Read the model definition and answer for the solid it produces. Units are mm, in the model's axes. A direction names the side the tool comes from. Give positions to 0.01 mm unless a question says otherwise; leave off trailing zeros. Order: outer loops, then holes, each group sorted by start corner. A loop starts at its lowest first (then second) coordinate and runs counter-clockwise, first axis right, second up.
Item 1: A cutting plane is placed at A-A (y = 3.75). Write down the section's boundary in (x, z).
Item 2: Which of the six approach directions +Z, -Z, +X, -X, +Y, -Y give full straight-line access (tool end or side, diameter ignored) to faces 1 (the face through (5, 3, 3.6)), 2 (the face through (5, 12, 1))?
Item 3: The mould has two halves that part along X. Classify faces 3 (the face through (3.92, 2.96, 2.85)), 4 (the face through (0, 6.9, 0.6)), 5 (the face through (10.4, 6.9, 0.6)), 6 (the face through (8, 3, 3.6)): +X half, -X half, draft (parallel to the pull), parting line (faces both ways), or undercut.
Item 4: A cutting plane is placed at B-B (x = 9.1). Write down the section's boundary in (y, z), plus the area to 3 significant figures.
Item 5: Given pin 1 Ø3 at (x, y) = (2.5, 14.5) entering from +Z, flat-ended and moving along its own axis, determine where the tip first touches the part or whether it passes through.
Item 6: A cutting plane is placed at C-C (x = 4.25). Write down the section's boundary in (y, z), plus the area to 3 significant figures.
Item 7: Find the intervals of material crossed by line 1 along Y through (x, z) = (0.5, 1.3); line 2 along Z through (x, y) = (3, 13.75); line 3 along X through (y, z) = (2.75, 3.3), in increasing order.
Item 8: A cutting plane is placed at D-D (y = 9.75). Write down the section's boundary in (x, z).
from build123d import *

# Parameters (mm, degrees)
BOX023_W          = 30
BOX023_H          = 20
BOX023_DEPTH      = 9.2
BOX007_W          = 26
BOX007_H          = 12
BOX007_DEPTH      = 5.2
CYLINDER002_R     = 0.75
CYLINDER002_DEPTH = 7
ARRAY002_X_COUNT  = 4
ARRAY002_X_PITCH  = 2.6
ARRAY002_Y_COUNT  = 2
ARRAY002_Y_PITCH  = 1
BOX_W             = 10.4
BOX_H             = 18
BOX_DEPTH         = 7.2


with BuildPart() as obj1:
    # Box023 → Box023 (new body)
    with BuildSketch(Plane(origin=(-1, -2, 3.6), x_dir=(1, 0, 0), z_dir=(0, 0, 1))):
        with Locations((15, 10)):
            Rectangle(BOX023_W, BOX023_H)
    extrude(amount=BOX023_DEPTH)


with BuildPart() as cube_10_base004:
    # Box007 → Box007 (new body)
    with BuildSketch(Plane(origin=(0, 6, 1), x_dir=(1, 0, 0), z_dir=(0, 0, 1))):
        with Locations((13, 6)):
            Rectangle(BOX007_W, BOX007_H)
    extrude(amount=BOX007_DEPTH)


with BuildPart() as array002:
    # Cylinder002 → Cylinder002 (new body)
    with BuildSketch(Plane(origin=(1.3, -1, 3.6), x_dir=(1, 0, 0), z_dir=(0, 1, 0))):
        Circle(CYLINDER002_R)
    extrude(amount=CYLINDER002_DEPTH)

    # Array002 X: Array002 ×4


with BuildPart() as array002_1:
    add(array002.part)
    with Locations(*[(i * ARRAY002_X_PITCH, 0, 0) for i in range(1, ARRAY002_X_COUNT)]):
        add(array002.part)

    # Array002 Y: Array002 ×2


with BuildPart() as array002_2:
    add(array002_1.part)
    with Locations(*[(0, i * ARRAY002_Y_PITCH, 0) for i in range(1, ARRAY002_Y_COUNT)]):
        add(array002_1.part)


with BuildPart() as obj2:
    # Box → Box (new body)
    with BuildSketch(Plane.XY):
        with Locations((5.2, 9)):
            Rectangle(BOX_W, BOX_H)
    extrude(amount=BOX_DEPTH)

    # Cut002: cut Array002
    add(array002_2.part, mode=Mode.SUBTRACT)

    # Cut006: cut cube_10_base004
    add(cube_10_base004.part, mode=Mode.SUBTRACT)

    # Cut019: cut obj1
    add(obj1.part, mode=Mode.SUBTRACT)


solid = obj2.part
Response values:
1. outline: (0, 0) - (10.4, 0) - (10.4, 3.6) - (9.85, 3.6) arc R0.75 cw to (8.35, 3.6) - (7.25, 3.6) arc R0.75 cw to (5.75, 3.6) - (4.65, 3.6) arc R0.75 cw to (3.15, 3.6) - (2.05, 3.6) arc R0.75 cw to (0.55, 3.6) - (0, 3.6) - close
2. face 1: +Z, +X, -X, +Y, -Y
2. face 2: +Z, +X, -X, +Y
3. face 3: undercut
3. face 4: -X half
3. face 5: +X half
3. face 6: draft
4. outline: (0, 0) - (18, 0) - (18, 1) - (6, 1) - (6, 2.85) - (0, 2.85) - close
4. area: 29.1 mm2
5. pin 1: stops at z = 1
6. outline: (0, 0) - (18, 0) - (18, 1) - (6, 1) - (6, 2.94) - (0, 2.94) - close
6. area: 29.6 mm2
7. line 1: y = 0 to 6
7. line 2: z = 0 to 1
7. line 3: x = 0 to 0.61, 1.99 to 3.21, 4.59 to 5.81, 7.19 to 8.41, 9.79 to 10.4
8. outline: (0, 0) - (10.4, 0) - (10.4, 1) - (0, 1) - close
